```python
from build123d import *

# Parameters (mm, degrees)
ESBO_O1_W                     = 72
ESBO_O1_H                     = 80
RESSALTO_EXTRUS_O1_DEPTH      = 30
ESBO_O3_W                     = 68
ESBO_O3_H                     = 76
CORTE_EXTRUS_O1_DEPTH         = 25
ESBO_O7_R                     = 10.25
RESSALTO_EXTRUS_O3_DEPTH      = 15
FILETE1_R                     = 4
RESSALTO_EXTRUS_O4_DEPTH      = 15
RESSALTO_EXTRUS_O4_DEPTH_BACK = 15
ESBO_O9_R                     = 18
ESBO_O10_R                    = 16.5
CORTE_EXTRUS_O2_DEPTH         = 40
RESSALTO_EXTRUS_O5_DEPTH      = 15
RESSALTO_EXTRUS_O5_DEPTH_BACK = 15
ESBO_O12_W                    = 17
ESBO_O12_H                    = 2
CORTE_EXTRUS_O3_DEPTH         = 40
FILETE2_R                     = 0.5
FILETE3_R                     = 0.5


with BuildPart() as part:
    # Esboço1 → Ressalto-extrusão1 (new body)
    with BuildSketch(Plane.XY):
        Rectangle(ESBO_O1_W, ESBO_O1_H)
    extrude(amount=RESSALTO_EXTRUS_O1_DEPTH)

    # Esboço3 → Corte-extrusão1 (cut)
    with BuildSketch(Plane.XY.offset(30)):
        Rectangle(ESBO_O3_W, ESBO_O3_H)
    extrude(amount=-CORTE_EXTRUS_O1_DEPTH, mode=Mode.SUBTRACT)

    # Esboço7 → Ressalto-extrusão3 (add)
    with BuildSketch(Plane(origin=(0, 0, 0), x_dir=(-1, 0, 0), z_dir=(0, 0, -1))):
        Circle(ESBO_O7_R)
    extrude(amount=RESSALTO_EXTRUS_O3_DEPTH)

    # Filete1
    filete1_edges = [part.edges().sort_by_distance(p)[0] for p in [
        (10.25, 0, 0),
    ]]
    fillet(filete1_edges, radius=FILETE1_R)

    # Esboço9 → Ressalto-extrusão4 (add, two sides: drawn at the far end of the back side and taken through both)
    with BuildSketch(Plane(origin=(0, 0, 0), x_dir=(0, 0, -1), z_dir=(1, 0, 0)).offset(-RESSALTO_EXTRUS_O4_DEPTH_BACK)):
        with Locations((27.479364999, 0)):
            Circle(ESBO_O9_R)
    extrude(amount=RESSALTO_EXTRUS_O4_DEPTH + RESSALTO_EXTRUS_O4_DEPTH_BACK)

    # Esboço10 → Corte-extrusão2 (cut)
    with BuildSketch(Plane(origin=(15, 0, 0), x_dir=(0, 0, -1), z_dir=(1, 0, 0))):
        with Locations((27.479364999, 0)):
            Circle(ESBO_O10_R)
    extrude(amount=-CORTE_EXTRUS_O2_DEPTH, mode=Mode.SUBTRACT)

    # Esboço11 → Ressalto-extrusão5 (add, two sides: drawn at the far end of the back side and taken through both)
    with BuildSketch(Plane(origin=(0, 0, 0), x_dir=(0, 0, -1), z_dir=(1, 0, 0)).offset(-RESSALTO_EXTRUS_O5_DEPTH_BACK)):
        Polygon((60.492568737, 0), (60.492568737, 4), (45.029293774, 4), (45.029293774, -4), (60.492568737, -4), align=None)
    extrude(amount=RESSALTO_EXTRUS_O5_DEPTH + RESSALTO_EXTRUS_O5_DEPTH_BACK)

    # Esboço12 → Corte-extrusão3 (cut)
    with BuildSketch(Plane(origin=(15, 0, 0), x_dir=(0, 0, -1), z_dir=(1, 0, 0))):
        with Locations((51.992568737, 1)):
            Rectangle(ESBO_O12_W, ESBO_O12_H)
    extrude(amount=-CORTE_EXTRUS_O3_DEPTH, mode=Mode.SUBTRACT)

    # Filete2
    filete2_edges = [part.edges().sort_by_distance(p)[0] for p in [
        (15, -1.001848456, -11.009808245),
    ]]
    fillet(filete2_edges, radius=FILETE2_R)

    # Filete3
    filete3_edges = [part.edges().sort_by_distance(p)[0] for p in [
        (-15, -1.001848456, -11.009808245),
    ]]
    fillet(filete3_edges, radius=FILETE3_R)


solid = part.part
```
Design review of the part built by this model. Coordinates are the model's own, in mm. A direction names the side the tool comes from. Round coordinates to 2 decimals unless told otherwise and drop trailing zeros. Order: outer loops, then holes, each group sorted by start corner. A loop starts at its lowest first (then second) coordinate and runs counter-clockwise, first axis right, second up. Notation, with made-up numbers: M 85.5,20 L 140.5,20 A28 cw 140.5,56 Z; hole C -4.75,63 d4. An arc over 180 degrees is marked long. Put each result on its own line as item: value.
Q1. To check wall thickness, follow line 1 (Y direction, x = 29, z = 12.5); line 2 (X direction, y = -19, z = 6); line 3 (Z direction, x = -14.5, y = 21.5). State the ranges of each line that lie inside material, in increasing order.
Reported:
line 1: -40 to -38, 38 to 40
line 2: -36 to -34, 34 to 36
line 3: 0 to 5
Q2. Consider section A-A (y = -20). State the section outline as (x, z) points.
Reported:
outline: M -36,0 L 36,0 L 36,30 L 34,30 L 34,5 L -34,5 L -34,30 L -36,30 Z
Q3. Draft analysis for pull direction X (two halves, no side actions). For faces 1 (the face through (36, -1, 15)), 2 (the face through (0, 1, 5)), 3 (the face through (-36, -1, 15)), 4 (the face through (0, 2, -52)), state which applies: released by +X, released by -X, zero draft, split by the parting line, or undercut.
Reported:
face 1: released by +X
face 2: undercut
face 3: released by -X
face 4: zero draft
Q4. Consider section B-B (z = -49.5). State the section outline as (x, y) points.
Reported:
outline: M -15,-4 L 15,-4 L 15,0 L -15,0 Z; M -15,2 L 15,2 L 15,4 L -15,4 Z
Q5. Machinability: for faces 5 (the face through (0, 0, -52)), 6 (the face through (10.24, 0.45, -7.32)), 7 (the face through (-15, -3.9, -44.3)), 8 (the face through (0, -4, -53)), 9 (the face through (-34, -1, 18)), which of the approach directions +Z, -Z, +X, -X, +Y, -Y give a long, thin tool a straight path to every point of the face, cutting with its end or side? Answer none if there is none.
Reported:
face 5: -Z, +X, -X
face 6: none
face 7: -Z, -X, +Y, -Y
face 8: -Z, +X, -X, -Y
face 9: +Z
Q6. Consider section D-D (x = 24.5). State the section outline as (y, z) points.
Reported:
outline: M -40,0 L 40,0 L 40,30 L 38,30 L 38,5 L -38,5 L -38,30 L -40,30 Z
Q7. Insertion check: pin 1 Ø6 at (x, y) = (-3.5, 17) entering from +Z; pin 2 Ø7.5 at (x, z) = (-5, -51) entering from -Y; pin 3 Ø4 at (y, z) = (-2.5, -3) entering from -X. Each pin has a flat end and moves straight along its axis. Give the tip position at first contact, or say it passes through.
Reported:
pin 1: z = 5
pin 2: y = -4
pin 3: x = -11.37
Q8. Consider section C-C (x = 0). State the section outline as (y, z) points.
Reported:
outline: M -40,0 L -14.25,0 A4 cw -10.25,-4 L -10.25,-12.68 A18 ccw -4,-45.03 L -4,-60.49 L 0,-60.49 L 0,-43.98 A16.5 cw long 2,-43.86 L 2,-60.49 L 4,-60.49 L 4,-45.03 A18 ccw 10.25,-12.68 L 10.25,-4 A4 cw 14.25,0 L 40,0 L 40,30 L 38,30 L 38,5 L -38,5 L -38,30 L -40,30 Z
